Read the model definition and answer for the solid it produces. Units are mm, in the model's axes. Face numbers are marked on the shaded views. A direction names the side the tool comes from. Round coordinates to 2 decimals unless told otherwise and drop trailing zeros. Write each loop counter-clockwise with the first axis right and the second up, starting at its lowest first coordinate (ties: lowest second). Pieces come first, ordered by that corner, then holes. Notation, with made-up numbers: (-16, 39.25) - (19, 39.25) arc R7 cw to (19, 51.25) - close; hole circle Ø11 at (-15.75, -11). An arc over 180 degrees is marked (long way). Answer as CSV lines item,"result". Start each with the question number.
1) Which of the six approach directions +Z, -Z, +X, -X, +Y, -Y give full straight-line access (tool end or side, diameter ignored) to the marked faces 4 and 5?
2) Find section D-D on y = 45. Determine the outline of the cut face in (x, z).
3) Each of these flat-tipped pins is pushed along its axis until it touches: pin 1 (12 mm diameter, centred on x = 17, y = 42.5, fed in from +Z); pin 2 (5 mm diameter, centred on x = 36.5, z = 5, fed in from +Y); pin 3 (20 mm diameter, centred on y = 19, z = 1.5, fed in from -X); pin 4 (8.5 mm diameter, centred on y = 48, z = -1.5, fed in from +X). Where does it stop, or does it pass through?
4) Consider line 1 along Y through (x, z) = (12.5, -8); line 2 along Y through (x, z) = (15, -5); line 3 along Y through (x, z) = (51, 14.5). Determine where each line is inside the solid, lowest interval first.
5) Find section C-C on x = 58. Determine the outline of the cut face in (y, z), then the cut area to 3 significant figures.
6) Find section A-A on y = 13. Determine the outline of the cut face in (x, z), then the cut area to 3 significant figures.
7) Find section B-B on z = -15.5. Determine the outline of the cut face in (x, y).
8) For a pull along Y with two mould halves and no side action, classify the marked faces 1, 2 and 3 as +Y half, -Y half, draft (parallel to the pull), parting line (faces both ways), or undercut.
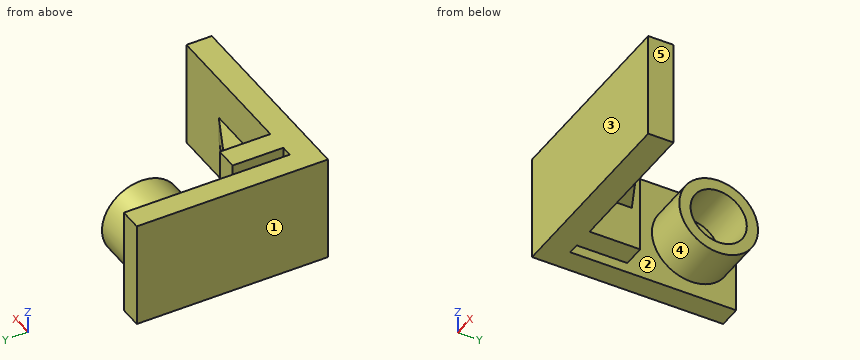
from build123d import *

# Parameters (mm, degrees)
SALIENTE_EXTRUIR2_DEPTH = 19
SALIENTE_EXTRUIR3_DEPTH = 32
CORTAR_EXTRUIR1_DEPTH   = 102.671038157
CROQUIS5_R              = 14
CROQUIS5_R_2            = 10
SALIENTE_EXTRUIR4_DEPTH = 17


with BuildPart() as part:
    # Croquis1 → Saliente-Extruir2 (new, symmetric)
    with BuildSketch(Plane.XY):
        Polygon((0, 0), (0, 68), (8, 68), (8, 9), (12, 9), (12, 27), (20, 27), (20, 9), (72, 9), (72, 0), align=None)
    extrude(amount=SALIENTE_EXTRUIR2_DEPTH, both=True)

    # Croquis3 → Saliente-Extruir3 (add)
    with BuildSketch(Plane(origin=(20, 0, 0), x_dir=(0, 0, -1), z_dir=(1, 0, 0))):
        Polygon((0, 9), (-4, 9), (-4, 24), (4, 24), (4, 9), align=None)
    extrude(amount=SALIENTE_EXTRUIR3_DEPTH)

    # Croquis4 → Cortar-Extruir1 (cut, through all)
    with BuildSketch(Plane.XY.offset(4)):
        Polygon((20, 24), (52, 9), (52, 24), align=None)
    extrude(amount=-CORTAR_EXTRUIR1_DEPTH, mode=Mode.SUBTRACT)

    # Croquis5 → Saliente-Extruir4 (add)
    with BuildSketch(Plane(origin=(8, 0, 0), x_dir=(0, 0, -1), z_dir=(1, 0, 0))):
        with Locations(Location((0, 52.035144158, 0), (0, 0, 270))):
            Circle(CROQUIS5_R)
        with Locations(Location((0, 52.035144158, 0), (0, 0, 90))):
            Circle(CROQUIS5_R_2, mode=Mode.SUBTRACT)
    extrude(amount=SALIENTE_EXTRUIR4_DEPTH)


solid = part.part
Check values:
1,face 4,"+X"
1,face 5,"+Z, -Z, +X, +Y, -Y"
2,outline,"(0, -19) - (8, -19) - (8, -12.1) - (25, -12.1) - (25, -7.11) - (8, -7.11) - (8, 7.11) - (25, 7.11) - (25, 12.1) - (8, 12.1) - (8, 19) - (0, 19) - close"
3,pin 1,"stops at z = 13.55"
3,pin 2,"stops at y = 17.34"
3,pin 3,"stops at x = 0"
3,pin 4,"stops at x = 8"
4,line 1,"y = 0 to 27, 40.55 to 46.04, 58.04 to 63.52"
4,line 2,"y = 0 to 27, 38.96 to 43.37, 60.7 to 65.11"
4,line 3,"y = 0 to 9"
5,outline,"(0, -19) - (9, -19) - (9, 19) - (0, 19) - close"
5,area,"342 mm^2"
6,outline,"(0, -19) - (8, -19) - (8, 19) - (0, 19) - close; (12, -19) - (20, -19) - (20, -4) - (43.47, -4) - (43.47, 4) - (20, 4) - (20, 19) - (12, 19) - close"
6,area,"796 mm^2"
7,outline,"(0, 0) - (72, 0) - (72, 9) - (20, 9) - (20, 27) - (12, 27) - (12, 9) - (8, 9) - (8, 68) - (0, 68) - close"
8,face 1,"draft"
8,face 2,"undercut"
8,face 3,"-Y half"
